CAD build for the part. Positions are in the model's coordinates, mm. A direction names the side the tool comes from. Round coordinates to 2 decimals unless told otherwise and drop trailing zeros.
Autodesk Inventor part; units mm, degrees
ref_plane "YZ Plane" through (0, 0, 0) normal (1, 0, 0) x (0, 1, 0)
ref_plane "XZ Plane" through (0, 0, 0) normal (0, 1, 0) x (-1, 0, 0)
ref_plane "XY Plane" through (0, 0, 0) normal (0, 0, 1) x (1, 0, 0)
sketch "Sketch1" plane through (0, 0, 0) normal (0, 0, 1) x (1, 0, 0)
  line L0 (0, 0) -> (152.4, 0)
  line L1 (152.4, 0) -> (152.4, 152.4)
  line L2 (152.4, 152.4) -> (0, 152.4)
  line L3 (0, 152.4) -> (0, 0)
  dimension "d0" = 152.4
  dimension "d1" = 152.4
extrude "Extrusion1" add sketch "Sketch1" along normal blind 6.35
sketch "Sketch2" plane through (0, 0, 6.35) normal (0, 0, 1) x (1, 0, 0)
  point P0 (0, 0)
  point P1 (15.24, 15.24)
  point P2 (45.72, 15.24)
  point P3 (76.2, 15.24)
  point P4 (106.68, 15.24)
  point P5 (137.16, 15.24)
  point P6 (15.24, 45.72)
  point P7 (45.72, 45.72)
  point P8 (76.2, 45.72)
  point P9 (106.68, 45.72)
  point P10 (137.16, 45.72)
  point P11 (137.16, 76.2)
  point P12 (106.68, 76.2)
  point P13 (76.2, 76.2)
  point P14 (45.72, 76.2)
  point P15 (15.24, 76.2)
  point P16 (15.24, 106.68)
  point P17 (45.72, 106.68)
  point P18 (76.2, 106.68)
  point P19 (106.68, 106.68)
  point P20 (137.16, 106.68)
  point P21 (137.16, 137.16)
  point P22 (106.68, 137.16)
  point P23 (76.2, 137.16)
  point P24 (45.72, 137.16)
  point P25 (15.24, 137.16)
hole "Hole1" at (15.24, 15.24, 6.35) at (45.72, 15.24, 6.35) at (76.2, 15.24, 6.35) at (106.68, 15.24, 6.35) at (137.16, 15.24, 6.35) at (15.24, 45.72, 6.35) at (45.72, 45.72, 6.35) at (76.2, 45.72, 6.35) at (106.68, 45.72, 6.35) at (137.16, 45.72, 6.35) at (137.16, 76.2, 6.35) at (106.68, 76.2, 6.35) at (76.2, 76.2, 6.35) at (45.72, 76.2, 6.35) at (15.24, 76.2, 6.35) at (15.24, 106.68, 6.35) at (45.72, 106.68, 6.35) at (76.2, 106.68, 6.35) at (106.68, 106.68, 6.35) at (137.16, 106.68, 6.35) at (137.16, 137.16, 6.35) at (106.68, 137.16, 6.35) at (76.2, 137.16, 6.35) at (45.72, 137.16, 6.35) at (15.24, 137.16, 6.35) direction (0, 0, -1) diameter 2.159 end through all
sketch "Sketch3" plane through (0, 0, 6.35) normal (0, 0, 1) x (1, 0, 0)
  line L0 (0, 0) -> (152.4, 0)
  line L1 (0, 152.4) -> (0, 0)
  point P0 (76.2, 25.4)
  point P1 (127, 25.4)
  point P2 (127, 127)
  point P3 (25.4, 25.8124)
  point P4 (50.8, 50.8)
  point P5 (127, 76.2)
  point P6 (101.6, 50.8)
  point P7 (50.8, 101.6)
  point P8 (25.4, 76.2)
  point P9 (25.4, 127)
  point P10 (76.2, 127)
  point P11 (101.6, 101.6)
  dimension "d19" = 25.4
  dimension "d21" = 25.4
  dimension "d23" = 25.4
  dimension "d25" = 76.2
  dimension "d27" = 127
  dimension "d28" = 76.2
  dimension "d30" = 127
  dimension "d33" = 50.8
  dimension "d38" = 50.8
  dimension "d40" = 101.6
  dimension "d42" = 50.8
  dimension "d43" = 50.8
  dimension "d46" = 25.4
  dimension "d48" = 25.4
  dimension "d55" = 50.8
  dimension "d56" = 101.6
hole "Hole2" at (76.2, 25.4, 6.35) at (127, 25.4, 6.35) at (127, 127, 6.35) at (25.4, 25.8124, 6.35) at (50.8, 50.8, 6.35) at (127, 76.2, 6.35) at (101.6, 50.8, 6.35) at (50.8, 101.6, 6.35) at (25.4, 76.2, 6.35) at (25.4, 127, 6.35) at (76.2, 127, 6.35) at (101.6, 101.6, 6.35) direction (0, 0, -1) diameter 6.35 end through all counterbore diameter 9.525 counterbore depth 3.302
ref_plane "Work Plane1" through (0, 76.2, 0) normal (0, 1, 0) x (1, 0, 0)
ref_plane "Work Plane2" through (76.2, 0, 0) normal (1, 0, 0) x (0, 0, -1)
properties part number "J010183" material "ALUMINUM, 6061-T651"
Item 1: Two-plate mould, pull along X, no slides. Class faces 1 (the cylindrical face through (22.25, 127.41, 1.5)), 2 (the flat face through (0, 77, 3)), 3 (the flat face through (75, 77, 6.35)): released by +X, released by -X, zero draft, split by the parting line, or undercut.
Answers follow:
face 1: undercut
face 2: released by -X
face 3: zero draft
Item 2: Cut at A-A, the plane y = 25.4. State how many separate pieces and enclosed holes the cut face has, plus the area to 3 significant figures.
Answers follow:
separate pieces: 4
enclosed holes: 0
area: 816 mm2
Item 3: Probe line 1 (X direction, y = 45.72, z = 2); line 2 (Y direction, x = 50.5, z = 2.75). List the from-to ranges inside material, lowest first.
Answers follow:
line 1: x = 0 to 14.16, 16.32 to 44.64, 46.8 to 75.12, 77.28 to 105.6, 107.76 to 136.08, 138.24 to 152.4
line 2: y = 0 to 47.64, 53.96 to 98.44, 104.76 to 152.4
Item 4: Flat gauge pin, fed straight in: P1, Ø8.5, axis at x = 25.4, y = 25.81, coming from the +Z side. Where does the tip first touch, or does it go through?
Answers follow:
P1: stops at z = 3.05
Item 5: 3-axis set-ups, long thin cutter, end or side, ignore diameter. For faces 4 (the cylindrical face through (105.825, 99.402, 4.676)), 5 (the cylindrical face through (23.25, 28.15, 1.5)): which of +Z, -Z, +X, -X, +Y, -Y reach the whole face in a straight line?
Answers follow:
face 4: +Z
face 5: +Z, -Z
